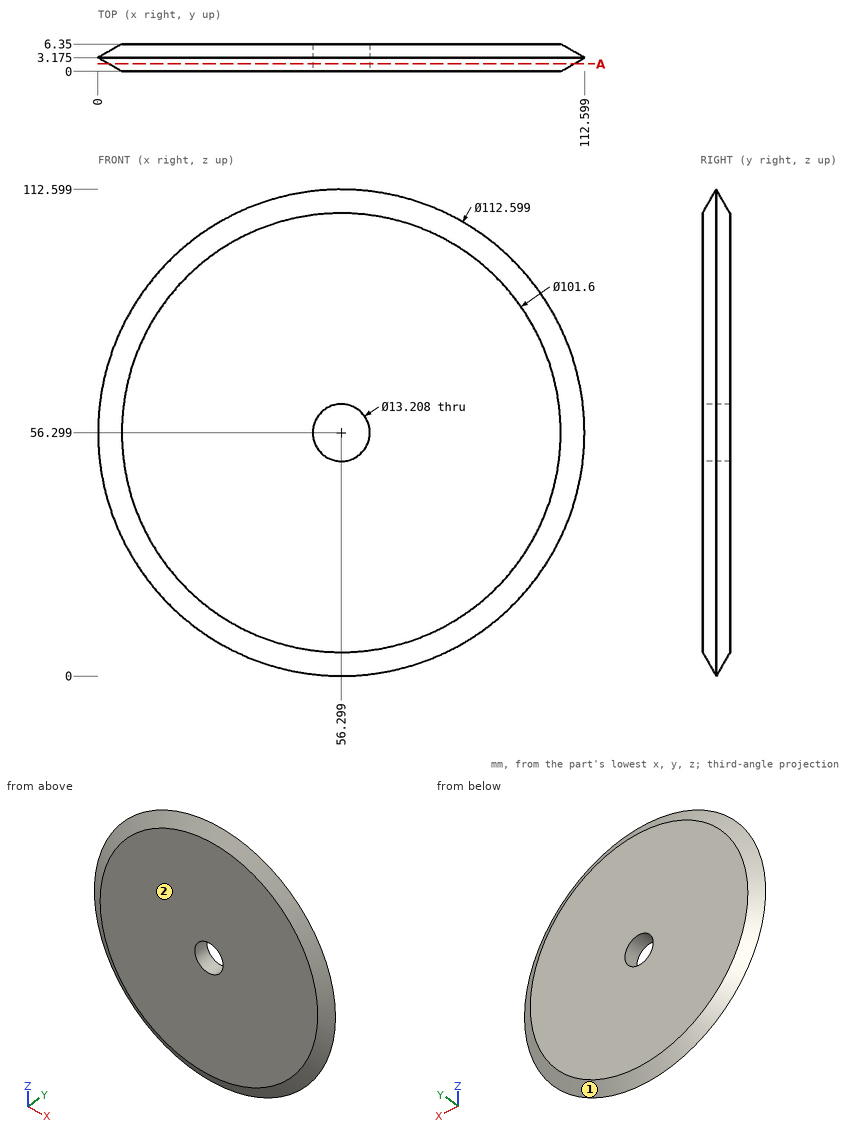
Verification items for this drawing (mm, ordinates from the low corner). Round coordinates to 2 decimals unless told otherwise and drop trailing zeros. Loops run counter-clockwise (first coordinate to the right, second up) from the corner with the lowest first, then second, coordinate; pieces in that order, holes last. Notation, with made-up numbers: (-7, 25) -> (39, 25) arc R13 cw to (39, 47) -> close; hole circle Ø3 at (81, 18). An arc over 180 degrees is marked (long way). Answer in a Markdown table with one row per item.
Q1. Go/stop test with a flat-tipped pin: P1, Ø1.5, axis at x = 50.5, y = 3.5, coming from the +Z side (1 decimal). Record where the tip stops, or that it passes through.
Data:
| item | result |
|---|---|
| P1 | stops at z = 112.4 |
Q2. Sectioned sample at A-A on y = 1.75. Enter the section's corners in (x, z) (1 decimal), then the cut area to 3 significant figures.
Data:
| item | result |
|---|---|
| outline | circle Ø107.7 at (56.3, 56.3); hole circle Ø13.2 at (56.3, 56.3) |
| area | 8,970 mm^2 |
Q3. Release check for a two-part mould opening along Y. For the marked faces 1 and 2 record: released by +Y, released by -Y, zero draft, split by the parting line, or undercut.
Data:
| item | result |
|---|---|
| face 1 | released by +Y |
| face 2 | released by -Y |
Q4. Thickness scan on L1, parallel to Z at x = 57.5, y = 1 (1 decimal); L2, parallel to X at y = 2.75, z = 59 (1 decimal); L3, parallel to X at y = 3.5, z = 72 (1 decimal). Record the ranges inside material, lowest first.
Data:
| item | result |
|---|---|
| L1 | z = 3.8 to 49.8, 62.8 to 108.8 |
| L2 | x = 0.8 to 50.3, 62.3 to 111.8 |
| L3 | x = 2.8 to 109.8 |
